Build history of the part. All positions in model axes, mm. A direction names the side the tool comes from. Give positions to 0.01 mm unless a question says otherwise; leave off trailing zeros. Loops run counter-clockwise (first coordinate to the right, second up) from the corner with the lowest first, then second, coordinate; pieces in that order, holes last. Notation, with made-up numbers: (88.25, 45) -> (146.25, 45) arc R12 cw to (146.25, 56) -> close; hole circle Ø11 at (29.5, -6). An arc over 180 degrees is marked (long way). Answer as a JSON object with one key per item and string values. Group by question number.
from build123d import *

# Parameters (mm, degrees)
BOX001_W     = 20
BOX001_H     = 30
BOX001_DEPTH = 34
BOX_W        = 20
BOX_H        = 24
BOX_DEPTH    = 38
BOX002_W     = 20
BOX002_H     = 8
BOX002_DEPTH = 8
BOX003_W     = 20
BOX003_H     = 10
BOX003_DEPTH = 10
FILLET_R     = 1


with BuildPart() as cube001:
    # Box001 → Box001 (new body)
    with BuildSketch(Plane(origin=(0, 2, 2), x_dir=(1, 0, 0), z_dir=(0, 0, 1))):
        with Locations((10, 15)):
            Rectangle(BOX001_W, BOX001_H)
    extrude(amount=BOX001_DEPTH)


with BuildPart() as cut:
    # Box → Box (new body)
    with BuildSketch(Plane.XY):
        with Locations((10, 12)):
            Rectangle(BOX_W, BOX_H)
    extrude(amount=BOX_DEPTH)

    # Cut: cut Cube001
    add(cube001.part, mode=Mode.SUBTRACT)


with BuildPart() as cube002:
    # Box002 → Box002 (new body)
    with BuildSketch(Plane(origin=(0, -8, 22), x_dir=(1, 0, 0), z_dir=(0, 0, 1))):
        with Locations((10, 4)):
            Rectangle(BOX002_W, BOX002_H)
    extrude(amount=BOX002_DEPTH)


with BuildPart() as fillet_body:
    # Box003 → Box003 (new body)
    with BuildSketch(Plane(origin=(0, -10, 20), x_dir=(1, 0, 0), z_dir=(0, 0, 1))):
        with Locations((10, 5)):
            Rectangle(BOX003_W, BOX003_H)
    extrude(amount=BOX003_DEPTH)

    # Cut001: cut Cube002
    add(cube002.part, mode=Mode.SUBTRACT)

    # Fusion: union Cut
    add(cut.part)

    # Fillet
    fillet_edges = [fillet_body.edges().sort_by_distance(p)[0] for p in [
        (10, -10, 30),
        (10, -10, 20),
        (10, 0, 0),
        (10, 0, 38),
        (10, 24, 38),
        (10, 24, 0),
    ]]
    fillet(fillet_edges, radius=FILLET_R)


solid = fillet_body.part
(1) Pull direction Y, two halves, no side cores. Call faces 1 (the flat face through (10, 12, 0)), 2 (the cylindrical face through (10.14, -9.699, 29.715)), 3 (the flat face through (10, 0, 29)): pulls with the +Y half, pulls with the -Y half, needs draft (parallel to the pull), parting line crosses it, or undercut.
(2) Saw through at A-A on y = 11.5. List the corners of the cut face in (x, z).
(3) Saw through at D-D on z = 5.5. List the corners of the cut face in (x, y).
(4) 3-axis set-ups, long thin cutter, end or side, ignore diameter. For faces 4 (the flat face through (10, -4, 20)), 5 (the flat face through (10, -8, 26)), 6 (the flat face through (9.9, -8.5, 30)), 7 (the flat face through (10, 2, 19)): which of +Z, -Z, +X, -X, +Y, -Y reach the whole face in a straight line?
(5) Saw through at B-B on z = 24.5. List the corners of the cut face in (x, y).
(6) Saw through at C-C on x = 16.5. List the corners of the cut face in (y, z), plus the area to 3 significant figures.
(7) Pin check, flat tips, straight feed: pin 1 (6.5 mm diameter, centred on x = 13, z = 27, fed in from +Y); pin 2 (2.5 mm diameter, centred on x = 12, y = -2.5, fed in from -Z); pin 3 (10 mm diameter, centred on x = 7.5, z = 12.5, fed in from -Y). Stop position of each tip, or through.
(8) Probe line 1 along Z through (x, y) = (10.25, 10); line 2 along Y through (x, z) = (17.5, 25.5); line 3 along Y through (x, z) = (2.75, 11). List the from-to ranges inside material, lowest first. Write a range as [from, to].
Calculated:
{
 "1": {"face 1": "needs draft", "face 2": "pulls with the -Y half", "face 3": "undercut"},
 "2": {"outline": "(0, 0) -> (20, 0) -> (20, 2) -> (0, 2) -> close; (0, 36) -> (20, 36) -> (20, 38) -> (0, 38) -> close"},
 "3": {"outline": "(0, 0) -> (20, 0) -> (20, 2) -> (0, 2) -> close"},
 "4": {"face 4": "-Z, +X, -X, -Y", "face 5": "+Z, +X, -X", "face 6": "+Z, +X, -X, -Y", "face 7": "+X, -X, +Y"},
 "5": {"outline": "(0, -10) -> (20, -10) -> (20, -8) -> (0, -8) -> close; (0, 0) -> (20, 0) -> (20, 2) -> (0, 2) -> close"},
 "6": {"outline": "(-10, 21) arc R1 ccw to (-9, 20) -> (0, 20) -> (0, 1) arc R1 ccw to (1, 0) -> (23, 0) arc R1 ccw to (24, 1) -> (24, 2) -> (2, 2) -> (2, 36) -> (24, 36) -> (24, 37) arc R1 ccw to (23, 38) -> (1, 38) arc R1 ccw to (0, 37) -> (0, 22) -> (-8, 22) -> (-8, 30) -> (-9, 30) arc R1 ccw to (-10, 29) -> close", "area": "199 mm^2"},
 "7": {"pin 1": "stops at y = 2", "pin 2": "stops at z = 20", "pin 3": "stops at y = 0"},
 "8": {"line 1": "z = [0, 2], [36, 38]", "line 2": "y = [-10, -8], [0, 2]", "line 3": "y = [0, 2]"}
}
